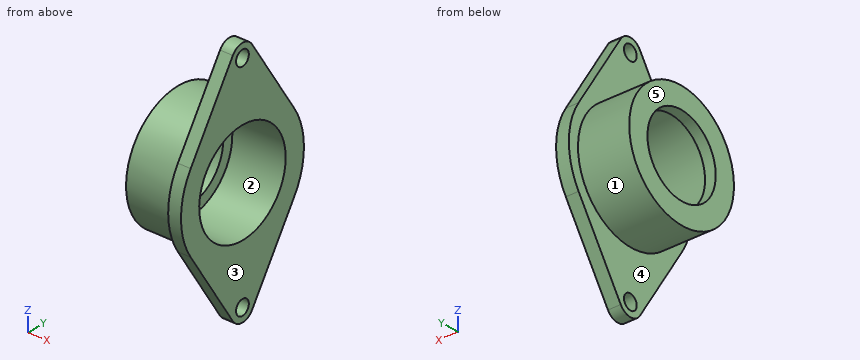
```python
from build123d import *

# Parameters (mm, degrees)
BOSS_EXTRUDE1_START = -12
SKETCH2_R           = 57.5
BOSS_EXTRUDE1_DEPTH = 12
SKETCH3_R           = 7
CUT_EXTRUDE1_DEPTH  = 12


with BuildPart() as part:
    # Sketch1 → Revolve1 (revolve)
    with BuildSketch(Plane.XY, mode=Mode.PRIVATE) as revolve1_sk:
        Polygon((-75.893975687, 34.641714336), (-25.893975687, 34.641714336), (-25.893975687, 44.641714336), (-85.893975687, 44.641714336), (-85.893975687, 24.641714336), (-75.893975687, 24.641714336), align=None)
    revolve(revolve1_sk.sketch.rotate(Axis((-85.893975687, -12.858285664, 0), (1, 0, 0)), 90), axis=Axis((-85.893975687, -12.858285664, 0), (1, 0, 0)))

    # Sketch2 → Boss-Extrude1 (add)
    with BuildSketch(Plane(origin=(-25.893975687, 0, 0), x_dir=(0, 0, -1), z_dir=(1, 0, 0)).offset(BOSS_EXTRUDE1_START)):
        with BuildLine():
            Line((36.425087952, -69.686649776), (109.207263185, -23.406395474))
            ThreePointArc((109.207263185, -23.406395474), (115, -12.858285664), (109.207263185, -2.310175853))
            Line((109.207263185, -2.310175853), (36.425087952, 43.970078449))
            ThreePointArc((36.425087952, 43.970078449), (0, 54.641714336), (-36.425087952, 43.970078449))
            Line((-36.425087952, 43.970078449), (-109.207263185, -2.310175853))
            ThreePointArc((-109.207263185, -2.310175853), (-115, -12.858285664), (-109.207263185, -23.406395474))
            Line((-109.207263185, -23.406395474), (-36.425087952, -69.686649776))
            ThreePointArc((-36.425087952, -69.686649776), (0, -80.358285664), (36.425087952, -69.686649776))
        make_face()
        with Locations(Location((0, -12.858285664, 0), (0, 0, 180))):
            Circle(SKETCH2_R, mode=Mode.SUBTRACT)
    extrude(amount=BOSS_EXTRUDE1_DEPTH)

    # Sketch3 → Cut-Extrude1 (cut)
    with BuildSketch(Plane(origin=(-25.893975687, 0, 0), x_dir=(0, 0, -1), z_dir=(1, 0, 0))):
        with Locations((-102.5, -12.858285664)):
            Circle(SKETCH3_R)
        with Locations((102.5, -12.858285664)):
            Circle(SKETCH3_R)
    extrude(amount=-CUT_EXTRUDE1_DEPTH, mode=Mode.SUBTRACT)


solid = part.part
```
Input: part model. Units: mm. Frame: model coordinates. Face numbers are marked on the shaded views. A direction names the side the tool comes from. Round coordinates to 2 decimals unless told otherwise and drop trailing zeros. Order: outer loops, then holes, each group sorted by start corner. A loop starts at its lowest first (then second) coordinate and runs counter-clockwise, first axis right, second up. Notation, with made-up numbers: (85.5, 66.5) - (129.5, 66.5) arc R17 ccw to (129.5, 96.5) - close; hole circle Ø8 at (-39.75, 53). An arc over 180 degrees is marked (long way). Answer in a Markdown table with one row per item.
Item 1: Section query A-A (z = 0). Return the cut outline in (x, y).
Model answer:
| item | result |
|---|---|
| outline | (-85.89, -70.36) - (-37.89, -70.36) - (-37.89, -80.36) - (-25.89, -80.36) - (-25.89, -60.36) - (-75.89, -60.36) - (-75.89, -50.36) - (-85.89, -50.36) - close; (-85.89, 24.64) - (-75.89, 24.64) - (-75.89, 34.64) - (-25.89, 34.64) - (-25.89, 54.64) - (-37.89, 54.64) - (-37.89, 44.64) - (-85.89, 44.64) - close |
Item 2: Pin query (flat end, axial travel): pin 1 (2 mm diameter, centred on x = -79, z = 8.5, fed in from -Y); pin 2 (1 mm diameter, centred on x = -35, y = -56.5, fed in from -Z); pin 3 (1.5 mm diameter, centred on x = -71.5, y = -36.5, fed in from -Z). Return the tip coordinate at first contact, or that it passes through.
Model answer:
| item | result |
|---|---|
| pin 1 | stops at y = -69.87 |
| pin 2 | stops at z = -57.95 |
| pin 3 | stops at z = -52.75 |
Item 3: Mould query, pull axis Z, two halves, no side actions, for the marked faces 1, 2 and 3. Classes: released by +Z, released by -Z, zero draft, split by the parting line, or undercut.
Model answer:
| item | result |
|---|---|
| face 1 | split by the parting line |
| face 2 | undercut |
| face 3 | zero draft |
Item 4: Section query D-D (z = 102.5). Return the cut outline in (x, y), then the cut area to 3 significant figures.
Model answer:
| item | result |
|---|---|
| outline | (-37.89, -27.67) - (-25.89, -27.67) - (-25.89, -19.86) - (-37.89, -19.86) - close; (-37.89, -5.86) - (-25.89, -5.86) - (-25.89, 1.95) - (-37.89, 1.95) - close |
| area | 188 mm² |
Item 5: Line query: line 1 (Y direction, x = -78.5, z = 0); line 2 (X direction, y = -71, z = -9); line 3 (Y direction, x = -31, z = -102). Output: solid intervals per line, ascending.
Model answer:
| item | result |
|---|---|
| line 1 | y = -70.36 to -50.36, 24.64 to 44.64 |
| line 2 | x = -37.89 to -25.89 |
| line 3 | y = -27.99 to -19.84, -5.88 to 2.27 |
Item 6: Reachability of the marked faces 4 and 5 from +Z, -Z, +X, -X, +Y, -Y: full face, straight path, thin tool, end or side. Return the list, or none.
Model answer:
| item | result |
|---|---|
| face 4 | -X |
| face 5 | +Z, -Z, -X, +Y, -Y |
Item 7: Section query B-B (y = -26.5). Return the cut outline in (x, z), then the cut area to 3 significant figures.
Model answer:
| item | result |
|---|---|
| outline | (-85.89, -55.86) - (-37.89, -55.86) - (-37.89, -104.34) - (-25.89, -104.34) - (-25.89, -45.5) - (-75.89, -45.5) - (-75.89, -34.93) - (-85.89, -34.93) - close; (-85.89, 34.93) - (-75.89, 34.93) - (-75.89, 45.5) - (-25.89, 45.5) - (-25.89, 104.34) - (-37.89, 104.34) - (-37.89, 55.86) - (-85.89, 55.86) - close |
| area | 2,620 mm² |
Item 8: Section query C-C (x = -81). Return the cut outline in (y, z), then the cut area to 3 significant figures.
Model answer:
| item | result |
|---|---|
| outline | circle Ø115 at (-12.86, 0); hole circle Ø75 at (-12.86, 0) |
| area | 5,970 mm² |
